Drawing for the job (mm, zero at the part's lowest x, y, z). Coordinates: 2 decimals unless noted, no trailing zeros. Loops run counter-clockwise (first coordinate to the right, second up) from the corner with the lowest first, then second, coordinate; pieces in that order, holes last. Notation, with made-up numbers: (69.5, 14.25) -> (100.5, 14.25) arc R22 ccw to (100.5, 33.25) -> close; hole circle Ø11 at (-25, 82). An arc over 180 degrees is marked (long way). Write each question's results on one line, items separated by ' | '.
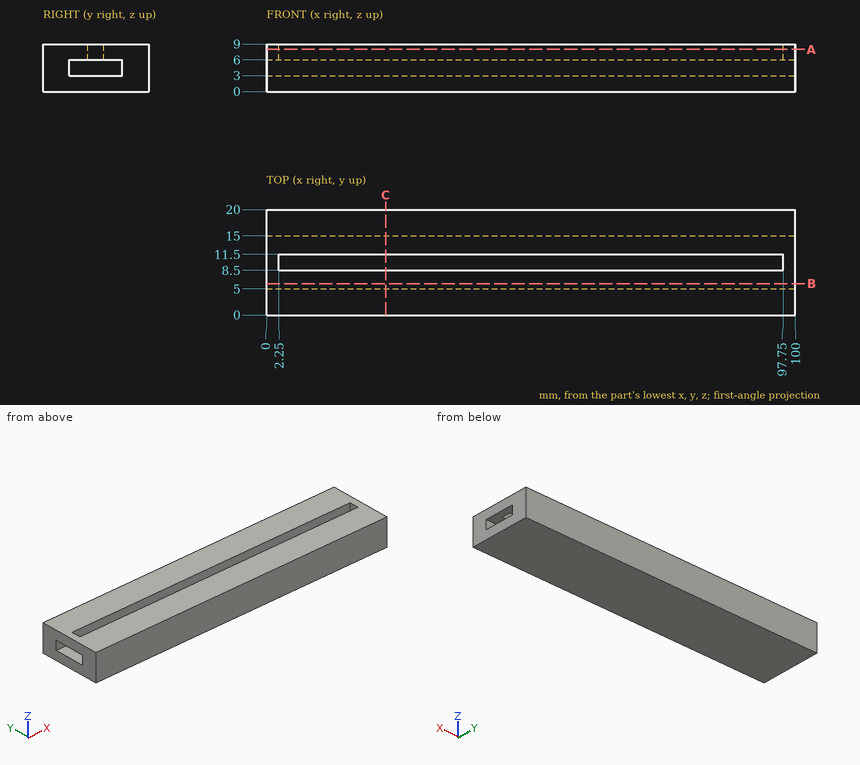
1) Slice it at B-B (y = 6). Write the cut outline in (x, z).
Outcome:
outline: (0, 0) -> (100, 0) -> (100, 3) -> (0, 3) -> close; (0, 6) -> (100, 6) -> (100, 9) -> (0, 9) -> close
2) Drill centre lines: L1, parallel to Y at x = 78.5, z = 7.5; L2, parallel to Z at x = 43, y = 14; L3, parallel to Y at x = 95, z = 5. Where is each one in solid material? Low to high. Write a range as from..to.
Outcome:
L1: y = 0..8.5, 11.5..20 | L2: z = 0..3, 6..9 | L3: y = 0..5, 15..20
3) Slice it at A-A (z = 8). Write the cut outline in (x, y).
Outcome:
outline: (0, 0) -> (100, 0) -> (100, 20) -> (0, 20) -> close; hole (2.25, 8.5) -> (97.75, 8.5) -> (97.75, 11.5) -> (2.25, 11.5) -> close
4) Slice it at C-C (x = 22.5). Write the cut outline in (y, z).
Outcome:
outline: (0, 0) -> (20, 0) -> (20, 9) -> (11.5, 9) -> (11.5, 6) -> (15, 6) -> (15, 3) -> (5, 3) -> (5, 6) -> (8.5, 6) -> (8.5, 9) -> (0, 9) -> close
5) Pin check, flat tip, straight feed: pin 1 (3 mm diameter, centred on y = 11, z = 7.5, fed in from -X). Stop position of the tip, or through.
Outcome:
pin 1: stops at x = 0
